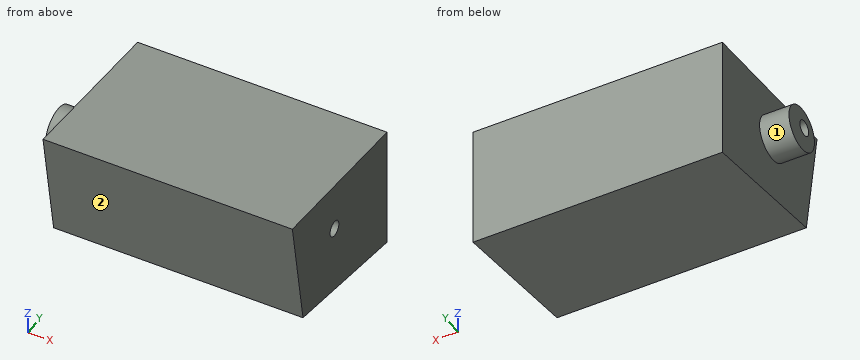
from build123d import *

# Parameters (mm, degrees)
F1_DEPTH = 101.346
F2_R     = 9.164769
F3_DEPTH = 113.284
F5_D     = 6.35


with BuildPart() as f1:
    # F0 (on Right) → F1 (new body)
    with BuildSketch(Plane.YZ):
        Polygon((18.714909, 17.103914), (-49.26987, 21.547778), (-41.631136, -24.609784), (18.714909, -33.40904), align=None)
    extrude(amount=F1_DEPTH)

    # F2 (on face) → F3 (join)
    with BuildSketch(Plane.YZ.offset(101.346)):
        with Locations((-17.187657, -1.531003)):
            Circle(F2_R)
    extrude(amount=-F3_DEPTH)

    # F5 (through all)
    with Locations(Plane(origin=(-11.938, 0, 0), x_dir=(0, -1, 0), z_dir=(-1, 0, 0))):
        with Locations((19.033102, 0)):
            Hole(F5_D / 2)


solid = f1.part
Could you check a few things on this model? Use its own coordinates, in mm. Face numbers are marked on the shaded views. A direction names the side the tool comes from. Round coordinates to 2 decimals unless told otherwise and drop trailing zeros. Order: outer loops, then holes, each group sorted by start corner. A loop starts at its lowest first (then second) coordinate and runs counter-clockwise, first axis right, second up.
Q1. Please list where these lines run through material, in increasing order: probe 1 along X at (y, z) = (-9.5, 7.5); probe 2 along Z at (x, y) = (43, -29); probe 3 along Z at (x, y) = (30, 4).
Geometry says:
probe 1: x = 0 to 101.35
probe 2: z = -26.45 to 20.22
probe 3: z = -31.26 to 18.07
Q2. Imagine slicing it at C-C, the plane z = 0. List the corners of the cut face in (x, y) for me, then the cut area to 3 significant figures.
Geometry says:
outline: (-11.94, -26.22) - (0, -26.22) - (0, -45.7) - (101.35, -45.7) - (101.35, -22.21) - (-11.94, -22.21) - close; (-11.94, -15.86) - (101.35, -15.86) - (101.35, 18.71) - (0, 18.71) - (0, -8.15) - (-11.94, -8.15) - close
area: 6,020 mm2
Q3. Imagine slicing it at D-D, the plane z = -8.5. List the corners of the cut face in (x, y) for me, then the cut area to 3 significant figures.
Geometry says:
outline: (-11.94, -23.14) - (0, -23.14) - (0, -44.3) - (101.35, -44.3) - (101.35, 18.71) - (0, 18.71) - (0, -11.24) - (-11.94, -11.24) - close
area: 6,530 mm2
Q4. Imagine slicing it at B-B, the plane y = -11. List the corners of the cut face in (x, z) for me.
Geometry says:
outline: (-11.94, -8.29) - (0, -8.29) - (0, -29.08) - (101.35, -29.08) - (101.35, 19.05) - (0, 19.05) - (0, 5.23) - (-11.94, 5.23) - close
Q5. Imagine slicing it at A-A, the plane x = 48. List the corners of the cut face in (y, z) for me (3 decimals).
Geometry says:
outline: (-49.27, 21.548) - (-41.631, -24.61) - (18.715, -33.409) - (18.715, 17.104) - close; hole circle Ø6.35 at (-19.033, 0)
Q6. I'm going to push flat-ended pins straight in: P1, Ø3, axis at x = 68.5, z = -8.5, coming from the -Y side; P2, Ø5, axis at x = 12, y = -4.5, coming from the +Z side; P3, Ø10, axis at x = 74.5, y = -26, coming from the +Z side. Where does each tip first touch, or does it pass through?
Geometry says:
P1: stops at y = -44.55
P2: stops at z = 18.78
P3: stops at z = 20.35
Q7. Which directions (+Z, -Z, +X, -X, +Y, -Y) give clear straight access to the entire face, cutting with the end or side of a thin tool? Please do the marked faces 1 and 2.
Geometry says:
face 1: -X
face 2: -Z, +X, -X, -Y
